Could you check a few things on this model? Use its own coordinates, in mm. A direction names the side the tool comes from. Coordinates: 2 decimals unless noted, no trailing zeros. Loops run counter-clockwise (first coordinate to the right, second up) from the corner with the lowest first, then second, coordinate; pieces in that order, holes last. Notation, with made-up numbers: (84.5, -36) - (104.5, -36) arc R34 cw to (104.5, -6) - close; hole circle Ø6 at (6.5, 35). An arc over 180 degrees is marked (long way). Use CSV: the item, a comma, the result in double quotes.
Autodesk Fusion 360 part; units mm, degrees
sketch "Skizze1" plane through (0, 0, 0) normal (0, 1, 0) x (1, 0, 0)
  arc A0 (0, 2) -> (2, 0) centre (2, 2) ccw
  arc A1 (2, 23) -> (0, 21) centre (2, 21) ccw
  line L0 (58.5, 23) -> (2, 23)
  line L1 (60.5, 2) -> (60.5, 21)
  arc A2 (58.5, 0) -> (60.5, 2) centre (58.5, 2) ccw
  line L2 (2, 0) -> (58.5, 0)
  line L3 (0, 21) -> (0, 2)
  arc A3 (60.5, 21) -> (58.5, 23) centre (58.5, 21) ccw
  point P0 (60.5, 0)
  point P1 (0, 23)
  dimension "d1" = 60.5
  dimension "d2" = 23
  dimension "d3" = 2
  dimension "d4" = 2
  dimension "d5" = 2
  dimension "d6" = 2
sketch "Skizze2" plane through (0, 0, 0) normal (0, 1, 0) x (1, 0, 0)
  line L0 (2.5, 1.5) -> (58, 1.5)
  line L1 (59, 2.5) -> (59, 20)
  line L2 (58, 21) -> (2.5, 21)
  line L3 (1.5, 20) -> (1.5, 2.5)
  line L4 (2, 0) -> (58.5, 0)
  line L5 (0, 21) -> (0, 2)
  arc A0 (2.5, 21) -> (1.5, 20) centre (2.5, 20) ccw
  arc A1 (1.5, 2.5) -> (2.5, 1.5) centre (2.5, 2.5) ccw
  arc A2 (59, 20) -> (58, 21) centre (58, 20) ccw
  arc A3 (58, 1.5) -> (59, 2.5) centre (58, 2.5) ccw
  point P0 (1.5, 1.5)
  point P1 (59, 1.5)
  point P2 (1.5, 21)
  dimension "d7" = 57.5
  dimension "d8" = 19.5
  dimension "d9" = 1.5
  dimension "d10" = 1.5
  dimension "d11" = 1
sketch "Skizze5" plane through (0, 0, 0) normal (0, 1, 0) x (1, 0, 0)
  line L0 (4, 4.2) -> (28, 4.2)
  line L1 (28, 4.2) -> (28, 18.8)
  line L2 (28, 18.8) -> (4, 18.8)
  line L3 (4, 18.8) -> (4, 4.2)
  line L4 (7.65, 7.5) -> (24.35, 7.5)
  line L5 (24.35, 7.5) -> (24.35, 15.5)
  line L6 (24.35, 15.5) -> (7.65, 15.5)
  line L7 (7.65, 15.5) -> (7.65, 7.5)
  line L8 (0, 21) -> (0, 2)
  line L9 (35.45, 7.5) -> (52.15, 7.5)
  line L10 (52.15, 15.5) -> (35.45, 15.5)
  line L11 (35.45, 15.5) -> (35.45, 7.5)
  line L12 (55.8, 4.2) -> (55.8, 18.8)
  line L13 (55.8, 18.8) -> (31.8, 18.8)
  line L14 (31.8, 18.8) -> (31.8, 4.2)
  line L15 (31.8, 4.2) -> (55.8, 4.2)
  line L16 (2, 0) -> (58.5, 0)
  line L17 (52.15, 7.5) -> (52.15, 15.5)
  dimension "d52" = 24
  dimension "d53" = 14.6
  dimension "d54" = 16.7
  dimension "d55" = 8
  dimension "d56" = 3.3
  dimension "d57" = 3.65
  dimension "d58" = 4
  dimension "d59" = 24
  dimension "d60" = 14.6
  dimension "d61" = 16.7
  dimension "d62" = 8
  dimension "d63" = 3.3
  dimension "d65" = 4.2
  dimension "d66" = 4.2
  dimension "d81" = 3.65
extrude "Extrusion8" add sketch "Skizze1" along normal blind 1.6
extrude "Extrusion9" add sketch "Skizze2" along normal blind 3.6
extrude "Extrusion10" cut sketch "Skizze5" along normal blind 20 contours L4 L5 L6 L7 | L9 L10 L11 L17
sketch "Skizze4" plane through (0, 0, 0) normal (0, 1, 0) x (1, 0, 0)
  circle A0 centre (44.5, 8) radius 1.5
  circle A1 centre (49.5, 8) radius 1.5
  circle A2 centre (54.5, 8) radius 1.5
  line L0 (2.5, 1.5) -> (58, 1.5)
  line L1 (24, 17.25) -> (24, 6.05)
  line L2 (36.5, 6.05) -> (36.5, 17.25)
  line L3 (2, 0) -> (58.5, 0)
  dimension "d16" = 3
  dimension "d17" = 3
  dimension "d18" = 3
  dimension "d19" = 5
  dimension "d20" = 5
  dimension "d25" = 8
  dimension "d26" = 8
extrude "Extrusion1" [suppressed]
extrude "Extrusion2" [suppressed]
extrude "Extrusion3" [suppressed]
equation "d16 = h1"
equation "d17 = h1"
equation "d18 = h1"
equation "h1 = 3 mm"
equation "h1_hoehe = 6.5 mm"
equation "d26 = h1_hoehe + ( h1 / 2 )"
(1) Suppose I cut it at B-B (y = 2.55). Write out the boundary of the cut face in (x, z).
Computed:
outline,"(1.5, -20) arc R1 ccw to (2.5, -21) - (58, -21) arc R1 ccw to (59, -20) - (59, -2.5) arc R1 ccw to (58, -1.5) - (2.5, -1.5) arc R1 ccw to (1.5, -2.5) - close; hole (7.65, -15.5) - (24.35, -15.5) - (24.35, -7.5) - (7.65, -7.5) - close; hole (35.45, -15.5) - (52.15, -15.5) - (52.15, -7.5) - (35.45, -7.5) - close"
(2) Will these pins go through, and if not, where does the flat tip stop? pin 1 (0.6 mm diameter, centred on y = 3, z = -10, fed in from +X); pin 2 (1.6 mm diameter, centred on y = 2.5, z = -12, fed in from -X).
Computed:
pin 1,"stops at x = 59"
pin 2,"stops at x = 1.5"
(3) Which directions (+Z, -Z, +X, -X, +Y, -Y) give clear straight access to the entire face, cutting with the end or side of a thin tool? Please do faces 5 (the face through (58.715, 2.586, -1.801)), 6 (the face through (1.801, 2.586, -1.785)), 7 (the face through (59, 3, -11)), 8 (the face through (28, 1.6, -1)), 9 (the face through (24.35, 2, -11)).
Computed:
face 5,"+Z, +X, +Y"
face 6,"+Z, -X, +Y"
face 7,"+Z, -Z, +X, +Y"
face 8,"+Y"
face 9,"+Y, -Y"
(4) Please list where these lines run through material, in increasing order: line 1 (X direction, y = 0.4, z = -14.5); line 2 (X direction, y = 3.4, z = -14.5); line 3 (Z direction, x = 13, y = 3.2).
Computed:
line 1,"x = 0 to 7.65, 24.35 to 35.45, 52.15 to 60.5"
line 2,"x = 1.5 to 7.65, 24.35 to 35.45, 52.15 to 59"
line 3,"z = -21 to -15.5, -7.5 to -1.5"
(5) Thinking about a two-plate mould opening in Z: for faces 1 (the face through (31, 3, -21)), 2 (the face through (30, 3, -1.5)), 3 (the face through (35.45, 2, -12)), 4 (the face through (44, 2, -7.5)), which applies, +Z half, -Z half, draft (parallel to the pull), parting line (faces both ways), or undercut?
Computed:
face 1,"-Z half"
face 2,"+Z half"
face 3,"undercut"
face 4,"undercut"
(6) Suppose I cut it at C-C (x = 11). Write out the boundary of the cut face in (y, z).
Computed:
outline,"(0, -23) - (1.6, -23) - (1.6, -21) - (3.6, -21) - (3.6, -15.5) - (0, -15.5) - close; (0, -7.5) - (3.6, -7.5) - (3.6, -1.5) - (1.6, -1.5) - (1.6, 0) - (0, 0) - close"
(7) Suppose I cut it at A-A (z = -12.5). Write out the boundary of the cut face in (x, y).
Computed:
outline,"(0, 0) - (7.65, 0) - (7.65, 3.6) - (1.5, 3.6) - (1.5, 1.6) - (0, 1.6) - close; (24.35, 0) - (35.45, 0) - (35.45, 3.6) - (24.35, 3.6) - close; (52.15, 0) - (60.5, 0) - (60.5, 1.6) - (59, 1.6) - (59, 3.6) - (52.15, 3.6) - close"
(8) Suppose I cut it at D-D (x = 31.5). Write out the boundary of the cut face in (y, z).
Computed:
outline,"(0, -23) - (1.6, -23) - (1.6, -21) - (3.6, -21) - (3.6, -1.5) - (1.6, -1.5) - (1.6, 0) - (0, 0) - close"
